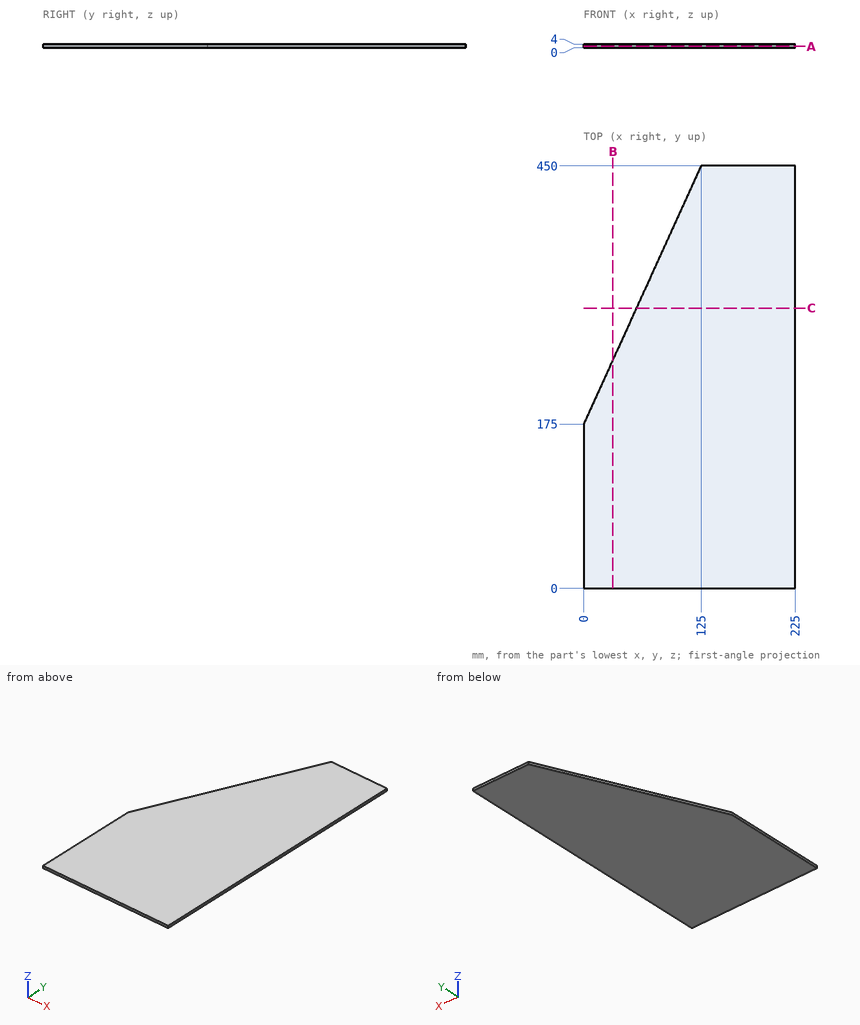
For this review, use the dimensioned drawing (mm, ordinates from the lowest corner) and the shaded views. Round coordinates to 2 decimals unless told otherwise and drop trailing zeros. Write each loop counter-clockwise with the first axis right and the second up, starting at its lowest first coordinate (ties: lowest second). Pieces come first, ordered by that corner, then holes. Notation, with made-up numbers: M 4,41 L 40,41 A27 ccw 40,79 Z; hole C 8,53 d4. An arc over 180 degrees is marked long. Write item = value, one per line. Start each with the question number.
(1) We need section A-A (z = 1.6). Give the boundary of the cut face in (x, y), then the cut area to 3 significant figures.
(2) For line 1 along Y through (x, z) = (22, 3.6); line 2 along Y through (x, z) = (29, 2.4); line 3 along X through (y, z) = (408, 3.1), list the stretches that pass through material, from the lowest coordinate up.
(3) We need section B-B (x = 31). Give the boundary of the cut face in (y, z).
(4) We need section C-C (y = 298.5). Give the boundary of the cut face in (x, z), then the cut area to 3 significant figures.
(5) Clearance check with a flat-ended pin moving along its axis: pin 1 Ø1 at (x, z) = (65.5, 1) entering from +Y. State where the tip first meets the part, or that it passes through.
Results found:
q1.outline = M 0,0 L 225,0 L 225,450 L 125,450 L 0,175 Z
q1.area = 84,100 mm²
q2.line_1 = 0 to 223.4
q2.line_2 = 0 to 238.8
q2.line_3 = 105.91 to 225
q3.outline = M 0,0 L 243.2,0 L 243.2,4 L 0,4 Z
q4.outline = M 56.14,0 L 225,0 L 225,4 L 56.14,4 Z
q4.area = 675 mm²
q5.pin_1 = 320.2
